Read the model definition and answer for the solid it produces. Units are mm, in the model's axes. A direction names the side the tool comes from. Give positions to 0.01 mm unless a question says otherwise; leave off trailing zeros. Write each loop counter-clockwise with the first axis right and the second up, starting at its lowest first coordinate (ties: lowest second). Pieces come first, ordered by that corner, then holes. Notation, with made-up numbers: M 0.5,31.25 L 53.5,31.25 A21 cw 53.5,65.25 Z; hole C -33.75,60.25 d11. An arc over 180 degrees is marked long. Put each result on its own line as item: value.
from build123d import *

# Parameters (mm, degrees)
SKETCH1_W           = 250
SKETCH1_H           = 125
SKETCH1_W_2         = 230
SKETCH1_H_2         = 115
BOSS_EXTRUDE1_DEPTH = 100
SKETCH3_W           = 250
SKETCH3_H           = 125
SKETCH3_W_2         = 230
SKETCH3_H_2         = 115
SKETCH3_R           = 20
SKETCH3_W_3         = 40
SKETCH3_H_3         = 40
BOSS_EXTRUDE4_DEPTH = 100


with BuildPart() as part:
    # Sketch1 → Boss-Extrude1 (new body)
    with BuildSketch(Plane.XY):
        Rectangle(SKETCH1_W, SKETCH1_H)
        Rectangle(SKETCH1_W_2, SKETCH1_H_2, mode=Mode.SUBTRACT)
    extrude(amount=BOSS_EXTRUDE1_DEPTH)

    # Sketch3 → Boss-Extrude4 (add)
    # profile 1 of 2: a face of its own
    with BuildSketch(Plane.XY.offset(100)):
        Rectangle(SKETCH3_W, SKETCH3_H)
        Rectangle(SKETCH3_W_2, SKETCH3_H_2, mode=Mode.SUBTRACT)
    # profile 2 of 2: a face of its own
    with BuildSketch(Plane.XY.offset(100)):
        Rectangle(SKETCH3_W_2, SKETCH3_H_2)
        with Locations((75, 0)):
            Circle(SKETCH3_R, mode=Mode.SUBTRACT)
        with Locations((-75, 0)):
            Rectangle(SKETCH3_W_3, SKETCH3_H_3, mode=Mode.SUBTRACT)
        Polygon((0, 23.094010768), (20, -11.547005384), (-20, -11.547005384), align=None, mode=Mode.SUBTRACT)
    extrude(amount=-BOSS_EXTRUDE4_DEPTH)


solid = part.part
(1) Section C-C on y = 0 is taken. Determine the outline of the cut face in (x, z), and give its area (3 significant figures).
Result:
outline: M -125,0 L -95,0 L -95,100 L -125,100 Z; M -55,0 L -13.33,0 L -13.33,100 L -55,100 Z; M 13.33,0 L 55,0 L 55,100 L 13.33,100 Z; M 95,0 L 125,0 L 125,100 L 95,100 Z
area: 14,300 mm²
(2) Section B-B on x = 75 is taken. Determine the outline of the cut face in (y, z).
Result:
outline: M -62.5,0 L -20,0 L -20,100 L -62.5,100 Z; M 20,0 L 62.5,0 L 62.5,100 L 20,100 Z
(3) Which of the six approach directions +Z, -Z, +X, -X, +Y, -Y give full straight-line access (tool end or side, diameter ignored) to faces 5 (the face through (-2, -13, 100)), 6 (the face through (-75, 20, 51))?
Result:
face 5: +Z, +X, -X, +Y, -Y
face 6: +Z, -Z
(4) Straight lines are drawn through the part: line 1 along Y through (x, z) = (75, 22); line 2 along X through (y, z) = (-16.5, 43.5); line 3 along X through (y, z) = (-4.5, 94). For each, find the intervals that lie inside material, in ascending order. Write a range as from..to.
Result:
line 1: y = -62.5..-20, 20..62.5
line 2: x = -125..-95, -55..63.7, 86.3..125
line 3: x = -125..-95, -55..-15.93, 15.93..55.51, 94.49..125
(5) Section A-A on z = 36.5 is taken. Determine the outline of the cut face in (x, y).
Result:
outline: M -125,-62.5 L 125,-62.5 L 125,62.5 L -125,62.5 Z; hole M -95,-20 L -55,-20 L -55,20 L -95,20 Z; hole M -20,-11.55 L 20,-11.55 L 0,23.09 Z; hole C 75,0 d40
(6) For a pull along X with two mould halves and no side action, classify faces 1 (the face through (-125, -1, 49)), 2 (the face through (-75, -20, 51)), 3 (the face through (9.86, 6.016, 50.7)), 4 (the face through (-2, 62.5, 49)) as +X half, -X half, draft (parallel to the pull), parting line (faces both ways), or undercut.
Result:
face 1: -X half
face 2: undercut
face 3: undercut
face 4: draft
